Verification items for the finished model (mm, model axes). Face numbers are marked on the shaded views. A direction names the side the tool comes from. Give positions to 0.01 mm unless a question says otherwise; leave off trailing zeros. Loops run counter-clockwise (first coordinate to the right, second up) from the corner with the lowest first, then second, coordinate; pieces in that order, holes last. Notation, with made-up numbers: (-37, 1.5) - (-2, 1.5) arc R30 cw to (-2, 27.5) - close; hole circle Ø9 at (-3, -7.5). An arc over 180 degrees is marked (long way). Answer in a Markdown table with one row per item.
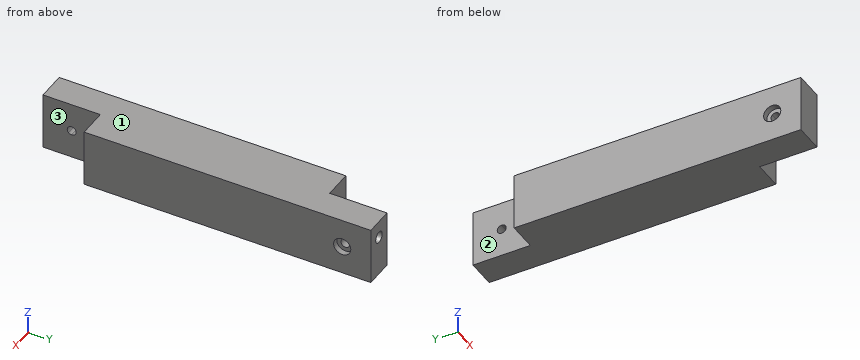
```python
from build123d import *

# Parameters (mm, degrees)
SKETCH_1_W          = 20
SKETCH_1_H          = 20
EXTRUDE_1_DEPTH     = 120
SKETCH_2_W          = 10
SKETCH_2_H          = 20
CUT_EXTRUDE_1_DEPTH = 120
SKETCH_3_W          = 10
SKETCH_3_H          = 20
CUT_EXTRUDE_2_DEPTH = 120
CUT_EXTRUDE_3_DEPTH = 120
SKETCH_5_R          = 3
CUT_EXTRUDE_4_DEPTH = 2
CUT_EXTRUDE_5_DEPTH = 20
SKETCH_7_R          = 3
CUT_EXTRUDE_6_DEPTH = 2
SKETCH_8_R          = 2
CUT_EXTRUDE_7_DEPTH = 100


with BuildPart() as part:
    # 草图1 → 凸台-拉伸1 (new body)
    with BuildSketch(Plane(origin=(0, 0, 0), x_dir=(1, 0, 0), z_dir=(0, 1, 0))):
        with Locations((-7.981321578, -6.453869679)):
            Rectangle(SKETCH_1_W, SKETCH_1_H)
    extrude(amount=EXTRUDE_1_DEPTH)

    # 草图2 → 切除-拉伸1 (cut)
    with BuildSketch(Plane.XY.offset(16.453869679)):
        with Locations((-12.981321578, 110)):
            Rectangle(SKETCH_2_W, SKETCH_2_H)
    extrude(amount=-CUT_EXTRUDE_1_DEPTH, mode=Mode.SUBTRACT)

    # 草图3 → 切除-拉伸2 (cut)
    with BuildSketch(Plane.XY.offset(16.453869679)):
        with Locations((-2.981321578, 10)):
            Rectangle(SKETCH_3_W, SKETCH_3_H)
    extrude(amount=-CUT_EXTRUDE_2_DEPTH, mode=Mode.SUBTRACT)

    # 草图4 → 切除-拉伸3 (cut)
    with BuildSketch(Plane.ZY.offset(7.981321578)):
        with BuildLine():
            ThreePointArc((8.003869679, 110), (7.047028999, 111.432013275), (5.357854168, 111.096015511))
            Line((5.357854168, 111.096015511), (7.549885189, 108.903984489))
            ThreePointArc((7.549885189, 108.903984489), (7.885882954, 109.40684068), (8.003869679, 110))
        make_face()
        with BuildLine():
            Line((7.549885189, 108.903984489), (5.357854168, 111.096015511))
            ThreePointArc((5.357854168, 111.096015511), (5.357854168, 108.903984489), (7.549885189, 108.903984489))
        make_face()
    extrude(amount=-CUT_EXTRUDE_3_DEPTH, mode=Mode.SUBTRACT)

    # 草图5 → 切除-拉伸4 (cut)
    with BuildSketch(Plane(origin=(2.018678422, 0, 0), x_dir=(0, 0, -1), z_dir=(1, 0, 0))):
        with Locations((-6.453869679, 110)):
            Circle(SKETCH_5_R)
    extrude(amount=-CUT_EXTRUDE_4_DEPTH, mode=Mode.SUBTRACT)

    # 草图6 → 切除-拉伸5 (cut)
    with BuildSketch(Plane(origin=(-7.981321578, 0, 0), x_dir=(0, 0, -1), z_dir=(1, 0, 0))):
        with BuildLine():
            ThreePointArc((-4.903869679, 10), (-5.860710358, 11.432013275), (-7.549885189, 11.096015511))
            Line((-7.549885189, 11.096015511), (-5.357854168, 8.903984489))
            ThreePointArc((-5.357854168, 8.903984489), (-5.021856403, 9.40684068), (-4.903869679, 10))
        make_face()
        with BuildLine():
            Line((-5.357854168, 8.903984489), (-7.549885189, 11.096015511))
            ThreePointArc((-7.549885189, 11.096015511), (-7.549885189, 8.903984489), (-5.357854168, 8.903984489))
        make_face()
    extrude(amount=-CUT_EXTRUDE_5_DEPTH, mode=Mode.SUBTRACT)

    # 草图7 → 切除-拉伸6 (cut)
    with BuildSketch(Plane.ZY.offset(17.981321578)):
        with Locations((6.453869679, 10)):
            Circle(SKETCH_7_R)
    extrude(amount=-CUT_EXTRUDE_6_DEPTH, mode=Mode.SUBTRACT)

    # 草图8 → 切除-拉伸7 (cut)
    with BuildSketch(Plane.XZ.offset(-20)):
        with Locations(Location((-2.981321578, 10.453869679, 0), (0, 0, 270))):
            Circle(SKETCH_8_R)
    extrude(amount=-CUT_EXTRUDE_7_DEPTH, mode=Mode.SUBTRACT)


solid = part.part
```
Q1. Thickness scan on line 1 (X direction, y = 15.5, z = 4.75); line 2 (Y direction, x = -17, z = 10.5); line 3 (Y direction, x = -10.25, z = 7.75). Record the ranges inside material, lowest first.
Completed:
| item | result |
|---|---|
| line 1 | -17.98 to -7.98 |
| line 2 | 0 to 100 |
| line 3 | 0 to 9.15, 10.85 to 100 |
Q2. Sectioned sample at B-B (z = -0.75). Record the cut outline in (x, y).
Completed:
| item | result |
|---|---|
| outline | (-17.98, 0) - (-7.98, 0) - (-7.98, 20) - (2.02, 20) - (2.02, 120) - (-7.98, 120) - (-7.98, 100) - (-17.98, 100) - close |
Q3. Tool access check on the marked faces 1, 2 and 3. Record the directions out of +Z, -Z, +X, -X, +Y, -Y that give a thin tool (end or side, any length) a straight path to the whole face; none if there is none.
Completed:
| item | result |
|---|---|
| face 1 | +Z, +X, -X, +Y, -Y |
| face 2 | +Z, -Z, -X, +Y |
| face 3 | +Z, -Z, +X, -Y |
Q4. Sectioned sample at A-A (x = -14.75). Record the cut outline in (y, z).
Completed:
| item | result |
|---|---|
| outline | (0, -3.55) - (100, -3.55) - (100, 16.45) - (0, 16.45) - close; hole circle Ø3.1 at (10, 6.45) |
Q5. Go/stop test with flat-tipped pins: P1, Ø6, axis at y = 13.5, z = 2.5, coming from the +X side; P2, Ø2, axis at x = -1.5, z = 5.5, coming from the -Y side; P3, Ø1, axis at x = -12, z = 4.5, coming from the -Y side; P4, Ø3.5, axis at y = 10, z = 6.45, coming from the -X side. Record where each tip stops, or that it passes through.
Completed:
| item | result |
|---|---|
| P1 | x = -7.98 |
| P2 | y = 20 |
| P3 | y = 0 |
| P4 | x = -15.98 |
Q6. Sectioned sample at C-C (y = 27). Record the cut outline in (x, z), and give its area (3 significant figures).
Completed:
| item | result |
|---|---|
| outline | (-17.98, -3.55) - (2.02, -3.55) - (2.02, 16.45) - (-17.98, 16.45) - close; hole circle Ø4 at (-2.98, 10.45) |
| area | 387 mm^2 |
